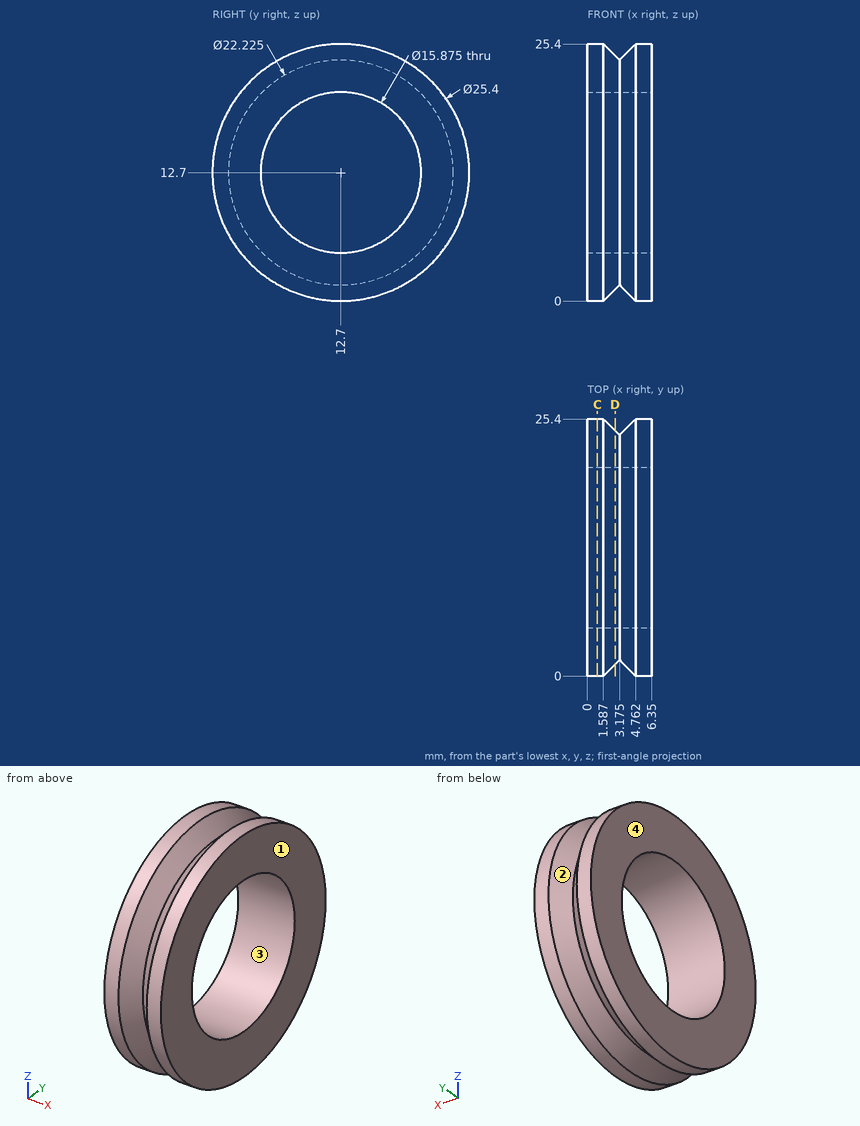
Here's the drawing with two shaded views (mm, measured from the low corner). I have some questions. Give positions to 0.01 mm unless a question says otherwise; leave off trailing zeros. Order: outer loops, then holes, each group sorted by start corner. A loop starts at its lowest first (then second) coordinate and runs counter-clockwise, first axis right, second up. Notation, with made-up numbers: (14, 89) -> (30, 89) arc R20 cw to (30, 125) -> close; hole circle Ø3 at (74, -9). An arc over 180 degrees is marked (long way). Use a Markdown table: item, result. Add a question column.
Item 1: Imagine slicing it at C-C on x = 1. Please give me the cut outline in (y, z) (1 decimal), plus the area to 3 significant figures.
Item 2: If we mould it in two halves opening along X, with no side actions, what happens to the marked faces 1, 2, 3 and 4? For each: pulls with the +X half, pulls with the -X half, needs draft (parallel to the pull), parting line crosses it, or undercut.
Item 3: I need wall thicknesses on line 1 (Z direction, x = 0.5, y = 16.25) (1 decimal); line 2 (X direction, y = 8, z = 23.5); line 3 (Z direction, x = 1, y = 9.75). Which ranges of each line are inside material? Lowest first, please.
Item 4: Imagine slicing it at D-D on x = 2.75. Please give me the cut outline in (y, z) (1 decimal).
Item 5: Will these pins go through, and if not, where does the flat tip stop? pin 1 (1 mm diameter, centred on x = 1, y = 22, fed in from -Z) (1 decimal); pin 2 (3 mm diameter, centred on x = 4, z = 23, fed in from +Y).
Data:
| question | item | result |
|---|---|---|
| 1 | outline | circle Ø25.4 at (12.7, 12.7); hole circle Ø15.9 at (12.7, 12.7) |
| 1 | area | 309 mm² |
| 2 | face 1 | pulls with the +X half |
| 2 | face 2 | undercut |
| 2 | face 3 | needs draft |
| 2 | face 4 | pulls with the -X half |
| 3 | line 1 | z = 0.5 to 5.6, 19.8 to 24.9 |
| 3 | line 2 | x = 0 to 2.51, 3.84 to 6.35 |
| 3 | line 3 | z = 0.35 to 5.33, 20.07 to 25.05 |
| 4 | outline | circle Ø23.1 at (12.7, 12.7); hole circle Ø15.9 at (12.7, 12.7) |
| 5 | pin 1 | stops at z = 3.5 |
| 5 | pin 2 | stops at y = 21.65 |
